from build123d import *

# Parameters (mm, degrees)
ESBO_O1_R                = 20.4
ESBO_O1_R_2              = 4.25
RESSALTO_EXTRUS_O1_DEPTH = 10
CORTE_EXTRUS_O1_DEPTH    = 4.5


with BuildPart() as part:
    # Esboço1 → Ressalto-extrusão1 (new body)
    with BuildSketch(Plane.XY):
        Circle(ESBO_O1_R)
        Circle(ESBO_O1_R_2, mode=Mode.SUBTRACT)
    extrude(amount=RESSALTO_EXTRUS_O1_DEPTH)

    # Esboço2 → Corte-extrusão1 (cut)
    with BuildSketch(Plane.XY.offset(10)):
        Polygon((3.810511777, -6.6), (7.621023553, 0), (3.810511777, 6.6), (-3.810511777, 6.6), (-7.621023553, 0), (-3.810511777, -6.6), align=None)
    extrude(amount=-CORTE_EXTRUS_O1_DEPTH, mode=Mode.SUBTRACT)


solid = part.part
Input: part model. Units: mm. Frame: model coordinates. A direction names the side the tool comes from. Coordinates: 2 decimals unless noted, no trailing zeros. Write each loop counter-clockwise with the first axis right and the second up, starting at its lowest first coordinate (ties: lowest second). Pieces come first, ordered by that corner, then holes. Notation, with made-up numbers: M -26,-20 L 0,-20 A17 ccw 0,-3 Z; hole C 26.5,16 d4. An arc over 180 degrees is marked long. Answer as a JSON object with one key per item and string values. Group by question number.
(1) Set-up query: faces 4 (the face through (3.3, 3, 5.5)), 5 (the face through (0, 5, 0)). Return all of +Z, -Z, +X, -X, +Y, -Y with unobstructed straight access to the full face (end or side cutting, diameter ignored); none if empty.
(2) Section D-D on y = -17. Output: boundary loops of the cut face in (x, z).
(3) Mould query, pull axis X, two halves, no side actions, for faces 1 (the face through (5.742, 3.254, 7.781)), 2 (the face through (9, 0, 10)), 3 (the face through (9.41, -18.1, 4.93)). Classes: pulls with the +X half, pulls with the -X half, needs draft (parallel to the pull), parting line crosses it, or undercut.
(4) Section A-A on x = 0. Output: boundary loops of the cut face in (y, z), plus the area to 3 significant figures.
(5) Section B-B on z = 6.25. Output: boundary loops of the cut face in (x, y), plus the area to 3 significant figures.
(6) Section C-C on x = 6. Output: boundary loops of the cut face in (y, z).
(7) Contact query for flat-ended pins moving along their axis: P1, Ø5, axis at x = 13, y = -0.5, coming from the -Z side; P2, Ø4, axis at x = 3, y = -2.5, coming from the +Z side; P3, Ø1.5, axis at y = 14, z = 7.5, coming from the -X side; P4, Ø2, axis at x = 1.5, z = 7.5, coming from the -Y side. Output: stop coordinate, or through.
(8) Ray query, line 1 along Y through (x, z) = (0, 3.8); line 2 along X through (y, z) = (1.5, 3); line 3 along X through (y, z) = (3, 9.75). Return the intervals inside material, ascending. Write a range as [from, to].
Result set:
{
 "1": {"face 4": "+Z", "face 5": "-Z, +X, -X, +Y, -Y"},
 "2": {"outline": "M -11.28,0 L 11.28,0 L 11.28,10 L -11.28,10 Z"},
 "3": {"face 1": "undercut", "face 2": "needs draft", "face 3": "parting line crosses it"},
 "4": {"outline": "M -20.4,0 L -4.25,0 L -4.25,5.5 L -6.6,5.5 L -6.6,10 L -20.4,10 Z; M 4.25,0 L 20.4,0 L 20.4,10 L 6.6,10 L 6.6,5.5 L 4.25,5.5 Z", "area": "302 mm2"},
 "5": {"outline": "C 0,0 d40.8; hole M -7.62,0 L -3.81,-6.6 L 3.81,-6.6 L 7.62,0 L 3.81,6.6 L -3.81,6.6 Z", "area": "1,160 mm2"},
 "6": {"outline": "M -19.5,0 L 19.5,0 L 19.5,10 L 2.81,10 L 2.81,5.5 L -2.81,5.5 L -2.81,10 L -19.5,10 Z"},
 "7": {"P1": "stops at z = 0", "P2": "stops at z = 5.5", "P3": "stops at x = -15.51", "P4": "stops at y = -20.39"},
 "8": {"line 1": "y = [-20.4, -4.25], [4.25, 20.4]", "line 2": "x = [-20.34, -3.98], [3.98, 20.34]", "line 3": "x = [-20.18, -5.89], [5.89, 20.18]"}
}
